```python
from build123d import *

# Parameters (mm, degrees)
BOSS_EXTRUDE1_DEPTH   = 24.13
SKETCH1_R             = 16.082263277
BOSS_EXTRUDE1_2_DEPTH = 24.13
SKETCH1_R_2           = 15.25707278
BOSS_EXTRUDE1_3_DEPTH = 24.13
SKETCH1_5_R           = 16.082263277
SKETCH1_5_R_2         = 15.25707278
BOSS_EXTRUDE2_DEPTH   = 6.096
BOSS_EXTRUDE3_DEPTH   = 6.096
CUT_EXTRUDE2_DEPTH    = 6.096
BOSS_EXTRUDE6_DEPTH   = 2.794
CUT_EXTRUDE3_DEPTH    = 0.762


with BuildPart() as part:
    # Sketch1 → Boss-Extrude1 (new body)
    with BuildSketch(Plane(origin=(0, 0, 0), x_dir=(1, 0, 0), z_dir=(0, 1, 0))):
        with BuildLine():
            ThreePointArc((-58.61646355, 0), (41.448098866, -41.448098866), (0, 58.61646355))
            ThreePointArc((0, 58.61646355), (-100.064562416, 100.064562416), (-58.61646355, 0))
        make_face()
        with BuildLine():
            ThreePointArc((-44.487942063, 0), (31.457725514, -31.457725514), (0, 44.487942063))
            Line((0, 44.487942063), (-14.199351912, 58.61646355))
            ThreePointArc((-14.199351912, 58.61646355), (-90.024104391, 90.024104391), (-58.61646355, 14.199351912))
            Line((-58.61646355, 14.199351912), (-44.487942063, 0))
        make_face(mode=Mode.SUBTRACT)
    extrude(amount=BOSS_EXTRUDE1_DEPTH)



with BuildPart() as body_2:
    # Sketch1 → Boss-Extrude1 2 (new body)
    with BuildSketch(Plane(origin=(0, 0, 0), x_dir=(1, 0, 0), z_dir=(0, 1, 0))):
        Circle(SKETCH1_R)
    extrude(amount=BOSS_EXTRUDE1_2_DEPTH)


with BuildPart() as body_3:
    # Sketch1 → Boss-Extrude1 3 (new body)
    with BuildSketch(Plane(origin=(0, 0, 0), x_dir=(1, 0, 0), z_dir=(0, 1, 0))):
        with Locations((-58.61646355, 58.61646355)):
            Circle(SKETCH1_R_2)
    extrude(amount=BOSS_EXTRUDE1_3_DEPTH)


with BuildPart() as part_1:
    add(part.part)

    add(body_2.part)  # Boss-Extrude2 merges body 2

    add(body_3.part)  # Boss-Extrude2 merges body 3
    # Sketch1_5 → Boss-Extrude2 (add)
    with BuildSketch(Plane(origin=(0, 0, 0), x_dir=(1, 0, 0), z_dir=(0, 1, 0))):
        with BuildLine():
            ThreePointArc((-58.61646355, 0), (41.448098866, -41.448098866), (0, 58.61646355))
            ThreePointArc((0, 58.61646355), (-100.064562416, 100.064562416), (-58.61646355, 0))
        make_face()
        with BuildLine():
            ThreePointArc((-44.487942063, 0), (31.457725514, -31.457725514), (0, 44.487942063))
            Line((0, 44.487942063), (-14.199351912, 58.61646355))
            ThreePointArc((-14.199351912, 58.61646355), (-90.024104391, 90.024104391), (-58.61646355, 14.199351912))
            Line((-58.61646355, 14.199351912), (-44.487942063, 0))
        make_face(mode=Mode.SUBTRACT)
        with BuildLine():
            Line((-44.487942063, 0), (-58.61646355, 14.199351912))
            ThreePointArc((-58.61646355, 14.199351912), (-90.024104391, 90.024104391), (-14.199351912, 58.61646355))
            Line((-14.199351912, 58.61646355), (0, 44.487942063))
            ThreePointArc((0, 44.487942063), (31.457725514, -31.457725514), (-44.487942063, 0))
        make_face()
        Circle(SKETCH1_5_R, mode=Mode.SUBTRACT)
        with Locations((-58.61646355, 58.61646355)):
            Circle(SKETCH1_5_R_2, mode=Mode.SUBTRACT)
        Circle(SKETCH1_5_R)
        with Locations((-58.61646355, 58.61646355)):
            Circle(SKETCH1_5_R_2)
    extrude(amount=-BOSS_EXTRUDE2_DEPTH)

    # Sketch5 → Boss-Extrude3 (add)
    with BuildSketch(Plane(origin=(0, 24.13, 0), x_dir=(1, 0, 0), z_dir=(0, 1, 0))):
        with BuildLine():
            Line((-114.656096447, 41.427823582), (-75.805103519, 2.576830654))
            ThreePointArc((-75.805103519, 2.576830654), (-100.064562416, 17.168364685), (-114.656096447, 41.427823582))
        make_face()
        with BuildLine():
            Line((17.188639969, 56.039632897), (56.039632897, 17.188639969))
            ThreePointArc((56.039632897, 17.188639969), (41.448098866, 41.448098866), (17.188639969, 56.039632897))
        make_face()
        with BuildLine():
            Line((-45.993671494, 115.704154646), (-2.576830654, 75.805103519))
            ThreePointArc((-2.576830654, 75.805103519), (-18.713405445, 101.817729032), (-45.993671494, 115.704154646))
        make_face()
        with BuildLine():
            Line((-17.188639969, -56.039632897), (-56.039632897, -17.188639969))
            ThreePointArc((-56.039632897, -17.188639969), (-41.448098866, -41.448098866), (-17.188639969, -56.039632897))
        make_face()
    extrude(amount=BOSS_EXTRUDE3_DEPTH)

    # Sketch6 → Cut-Extrude2 (cut)
    with BuildSketch(Plane(origin=(0, 24.13, 0), x_dir=(1, 0, 0), z_dir=(0, 1, 0))):
        with BuildLine():
            ThreePointArc((-9.489981352, 0), (-6.710430167, -6.710430167), (0, -9.489981352))
            ThreePointArc((0, -9.489981352), (5.668121673, -5.668121673), (9.489981352, 0))
            ThreePointArc((9.489981352, 0), (6.710430167, 6.710430167), (0, 9.489981352))
            ThreePointArc((0, 9.489981352), (-5.677482123, 5.677482123), (-9.489981352, 0))
        make_face()
        with BuildLine():
            ThreePointArc((-48.996622209, 58.61646355), (-51.814208504, 65.418718597), (-58.61646355, 68.236304892))
            ThreePointArc((-58.61646355, 68.236304892), (-64.379822748, 64.379822748), (-68.236304892, 58.61646355))
            ThreePointArc((-68.236304892, 58.61646355), (-65.418718597, 51.814208504), (-58.61646355, 48.996622209))
            ThreePointArc((-58.61646355, 48.996622209), (-52.847164261, 52.847164261), (-48.996622209, 58.61646355))
        make_face()
    extrude(amount=-CUT_EXTRUDE2_DEPTH, mode=Mode.SUBTRACT)

    # Sketch7 → Boss-Extrude6 (add)
    with BuildSketch(Plane(origin=(0, 24.13, 0), x_dir=(1, 0, 0), z_dir=(0, 1, 0))):
        with BuildLine():
            ThreePointArc((-55.830465051, 2.585437245), (39.520408105, -39.520408105), (-2.585437245, 55.830465051))
            ThreePointArc((-2.585437245, 55.830465051), (-98.285328524, 98.285328524), (-55.830465051, 2.585437245))
        make_face()
    extrude(amount=BOSS_EXTRUDE6_DEPTH)

    # Sketch7_3 → Cut-Extrude3 (cut)
    with BuildSketch(Plane(origin=(0, 24.13, 0), x_dir=(1, 0, 0), z_dir=(0, 1, 0))):
        with BuildLine():
            ThreePointArc((-55.830465051, 2.585437245), (39.520408105, -39.520408105), (-2.585437245, 55.830465051))
            ThreePointArc((-2.585437245, 55.830465051), (-98.285328524, 98.285328524), (-55.830465051, 2.585437245))
        make_face()
    extrude(amount=CUT_EXTRUDE3_DEPTH, mode=Mode.SUBTRACT)


solid = part_1.part
```
Design review of the part built by this model. Coordinates are the model's own, in mm. A direction names the side the tool comes from. Coordinates: 2 decimals unless noted, no trailing zeros. Write each loop counter-clockwise with the first axis right and the second up, starting at its lowest first coordinate (ties: lowest second). Pieces come first, ordered by that corner, then holes. Notation, with made-up numbers: M 16,56 L 46,56 A23 cw 46,73 Z; hole C 10.5,25.5 d11. An arc over 180 degrees is marked long. Answer as a JSON object with one key per item and string values.
Item 1: Add section D-D, the plane z = 38.5. Give the boundary of the cut face in (x, y), and give its area (3 significant figures).
Outcome:
{"outline": "M -44.2,-6.1 L 44.2,-6.1 L 44.2,24.13 L 22.29,24.13 L 22.29,0 L -22.29,0 L -22.29,24.13 L -40.52,24.13 L -40.52,24.89 L 40.52,24.89 L 40.52,26.92 L -34.73,26.92 L -34.73,30.23 L -44.2,30.23 Z", "area": "1,800 mm²"}
Item 2: Insertion check: pin 1 Ø2 at (x, y) = (31.5, 17) entering from +Z; pin 2 Ø12 at (y, z) = (26, 10) entering from +X; pin 3 Ø10 at (y, z) = (-1, -19) entering from +X. Each pin has a flat end and moves straight along its axis. Give the tip position at first contact, or say it passes through.
Outcome:
{"pin 1": "z = 50.06", "pin 2": "x = 58.46", "pin 3": "x = 56.92"}
Item 3: Add section A-A, the plane y = 21. Give the boundary of the cut face in (x, z).
Outcome:
{"outline": "C -58.62,-58.62 d30.51; M -58.62,0 A58.62 ccw long 0,-58.62 A58.62 ccw long Z; C 0,0 d32.16; hole M -68.24,-58.62 A17.83 ccw -58.62,-68.24 A9.62 ccw -49,-58.62 A17.73 ccw -58.62,-49 A9.62 ccw Z; hole M -58.62,-14.2 A44.42 ccw long -14.2,-58.62 L 0,-44.49 A44.49 ccw long -44.49,0 Z; hole M -9.49,0 A17.73 ccw 0,-9.49 A9.49 ccw 9.49,0 A17.9 ccw 0,9.49 A9.49 ccw Z"}
Item 4: Machinability: for faces 4 (the flat face through (-7, 11.896, -51.453)), 5 (the cylindrical face through (39.73, 24.51, -39.31)), 6 (the cylindrical face through (-20.398, 24.506, -99.685)), 7 (the cylindrical face through (-39.73, 24.51, 39.31)), which of the approach directions +Z, -Z, +X, -X, +Y, -Y give a long, thin tool a straight path to every point of the face, cutting with its end or side? Answer none if there is none.
Outcome:
{"face 4": "none", "face 5": "+Z", "face 6": "-X", "face 7": "+X"}
Item 5: Add section B-B, the plane y = 3. Give the boundary of the cut face in (x, z), and give its area (3 significant figures).
Outcome:
{"outline": "C -58.62,-58.62 d30.51; M -58.62,0 A58.62 ccw long 0,-58.62 A58.62 ccw long Z; C 0,0 d32.16; hole M -58.62,-14.2 A44.42 ccw long -14.2,-58.62 L 0,-44.49 A44.49 ccw long -44.49,0 Z", "area": "8,620 mm²"}
Item 6: Wall thickness on probe 1 along Y at (x, z) = (-16.5, 17); probe 2 along Y at (x, z) = (-92.5, -96.5); probe 3 along Z at (x, y) = (7.5, 9): over which ranges is each line inside the solid? List them lowest first.
Outcome:
{"probe 1": "-6.1 to 0, 24.89 to 26.92", "probe 2": "-6.1 to 24.13, 24.89 to 26.92", "probe 3": "-58.13 to -43.85, -14.23 to 14.23, 43.85 to 58.13"}
Item 7: Draft analysis for pull direction Y (two halves, no side actions). For faces 1 (the flat face through (-97, 30.226, -19)), 2 (the flat face through (-30, 0, -30)), 3 (the flat face through (-31, -6.096, -31)), state which applies: pulls with the +Y half, pulls with the -Y half, needs draft (parallel to the pull), parting line crosses it, or undercut.
Outcome:
{"face 1": "pulls with the +Y half", "face 2": "undercut", "face 3": "pulls with the -Y half"}
Item 8: Add section C-C, the plane x = -71.5. Give the boundary of the cut face in (y, z), and give its area (3 significant figures).
Outcome:
{"outline": "M -6.1,-115.8 L 24.13,-115.8 L 24.13,-101.12 L 0,-101.12 L 0,-66.79 L 24.13,-66.79 L 24.13,-50.44 L 0,-50.44 L 0,-16.11 L 24.13,-16.11 L 24.13,-1.43 L -6.1,-1.43 Z; M 24.89,-113.22 L 26.92,-113.22 L 26.92,-4.02 L 24.89,-4.02 Z", "area": "2,020 mm²"}
